from build123d import *

# Parameters (mm, degrees)
SKETCH1_W           = 109.86
SKETCH1_H           = 109.86
SKETCH1_R           = 4.25
BOSS_EXTRUDE1_DEPTH = 201
FILLET1_R           = 5
SKETCH2_R           = 27.6
BOSS_EXTRUDE2_DEPTH = 1.52
SKETCH3_R           = 9.5
BOSS_EXTRUDE3_DEPTH = 55.37
CUT_EXTRUDE1_START  = -12.5
CUT_EXTRUDE1_DEPTH  = 205.37
FILLET2_R           = 3


with BuildPart() as part:
    # Sketch1 → Boss-Extrude1 (new body)
    with BuildSketch(Plane(origin=(0, 0, 0), x_dir=(1, 0, 0), z_dir=(0, 1, 0))):
        Rectangle(SKETCH1_W, SKETCH1_H)
        with Locations(Location((-44.5, 44.5, 0), (0, 0, 270))):
            Circle(SKETCH1_R, mode=Mode.SUBTRACT)
        with Locations(Location((44.5, 44.5, 0), (0, 0, 270))):
            Circle(SKETCH1_R, mode=Mode.SUBTRACT)
        with Locations(Location((44.5, -44.5, 0), (0, 0, 270))):
            Circle(SKETCH1_R, mode=Mode.SUBTRACT)
        with Locations(Location((-44.5, -44.5, 0), (0, 0, 270))):
            Circle(SKETCH1_R, mode=Mode.SUBTRACT)
    extrude(amount=-BOSS_EXTRUDE1_DEPTH)

    # Fillet1
    fillet1_edges = [part.edges().sort_by_distance(p)[0] for p in [
        (54.93, -100.5, 54.93),
        (-54.93, -100.5, 54.93),
        (-54.93, -100.5, -54.93),
        (54.93, -100.5, -54.93),
    ]]
    fillet(fillet1_edges, radius=FILLET1_R)

    # Sketch2 → Boss-Extrude2 (add)
    with BuildSketch(Plane(origin=(0, 0, 0), x_dir=(1, 0, 0), z_dir=(0, 1, 0))):
        with Locations(Location((0, 0, 0), (0, 0, 90))):
            Circle(SKETCH2_R)
    extrude(amount=BOSS_EXTRUDE2_DEPTH)

    # Sketch3 → Boss-Extrude3 (add)
    with BuildSketch(Plane(origin=(0, 0, 0), x_dir=(1, 0, 0), z_dir=(0, 1, 0))):
        with Locations(Location((0, 0, 0), (0, 0, 270))):
            Circle(SKETCH3_R)
    extrude(amount=BOSS_EXTRUDE3_DEPTH)

    # Sketch5 → Cut-Extrude1 (cut)
    with BuildSketch(Plane(origin=(0, 0, 0), x_dir=(1, 0, 0), z_dir=(0, 1, 0)).offset(CUT_EXTRUDE1_START)):
        with BuildLine():
            Line((-44.5, 32.5), (-57.57926657, 32.5))
            Line((-57.57926657, 32.5), (-57.57926657, 62.356452686))
            Line((-57.57926657, 62.356452686), (-32.5, 61.861560204))
            Line((-32.5, 61.861560204), (-32.5, 44.5))
            ThreePointArc((-32.5, 44.5), (-36.014718626, 36.014718626), (-44.5, 32.5))
        make_face()
        with BuildLine():
            Line((62.356452686, 57.57926657), (61.861560204, 32.5))
            Line((61.861560204, 32.5), (44.5, 32.5))
            ThreePointArc((44.5, 32.5), (36.014718626, 36.014718626), (32.5, 44.5))
            Line((32.5, 44.5), (32.5, 57.57926657))
            Line((32.5, 57.57926657), (62.356452686, 57.57926657))
        make_face()
        with BuildLine():
            Line((57.57926657, -62.356452686), (32.5, -61.861560204))
            Line((32.5, -61.861560204), (32.5, -44.5))
            ThreePointArc((32.5, -44.5), (36.014718626, -36.014718626), (44.5, -32.5))
            Line((44.5, -32.5), (57.57926657, -32.5))
            Line((57.57926657, -32.5), (57.57926657, -62.356452686))
        make_face()
        with BuildLine():
            Line((-62.356452686, -57.57926657), (-61.861560204, -32.5))
            Line((-61.861560204, -32.5), (-44.5, -32.5))
            ThreePointArc((-44.5, -32.5), (-36.014718626, -36.014718626), (-32.5, -44.5))
            Line((-32.5, -44.5), (-32.5, -57.57926657))
            Line((-32.5, -57.57926657), (-62.356452686, -57.57926657))
        make_face()
    extrude(amount=-CUT_EXTRUDE1_DEPTH, mode=Mode.SUBTRACT)

    # Fillet2
    fillet2_edges = [part.edges().sort_by_distance(p)[0] for p in [
        (32.5, -106.75, 54.93),
        (32.5, -106.75, -54.93),
        (54.93, -106.75, -32.5),
        (-54.93, -106.75, -32.5),
        (-32.5, -106.75, -54.93),
        (-32.5, -106.75, 54.93),
        (-54.93, -106.75, 32.5),
        (54.93, -106.75, 32.5),
    ]]
    fillet(fillet2_edges, radius=FILLET2_R)


solid = part.part
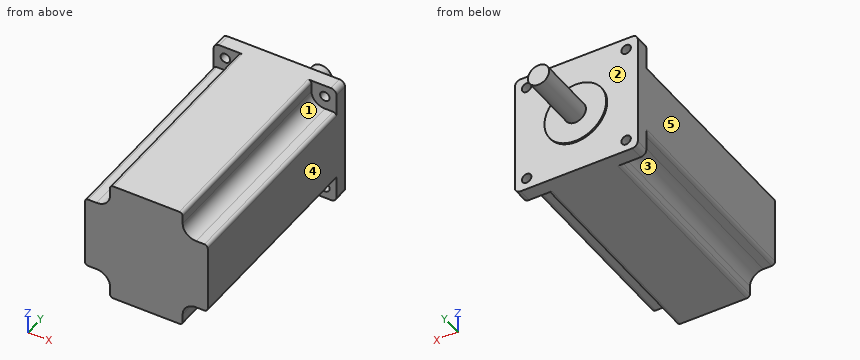
Geometry: final body of the model. Coordinates: model frame, mm. Face numbers are marked on the shaded views. A direction names the side the tool comes from. Coordinates: 2 decimals unless noted, no trailing zeros. Order: outer loops, then holes, each group sorted by start corner. A loop starts at its lowest first (then second) coordinate and runs counter-clockwise, first axis right, second up.
1) Section A-A (x = 0). Return loops of the section in (y, z).
Result sheet:
outline: (-201, -54.93) - (0, -54.93) - (0, -27.6) - (1.52, -27.6) - (1.52, -9.5) - (55.37, -9.5) - (55.37, 9.5) - (1.52, 9.5) - (1.52, 27.6) - (0, 27.6) - (0, 54.93) - (-201, 54.93) - close
2) Set-up query: the marked faces 1, 2, 3, 4 and 5. Return all of +Z, -Z, +X, -X, +Y, -Y with unobstructed straight access to the full face (end or side cutting, diameter ignored); none if empty.
Result sheet:
face 1: +Z, +X, -Y
face 2: +Y
face 3: -Z, -X, -Y
face 4: +Z, -Z, +X, +Y, -Y
face 5: +Z, -Z, -X, +Y, -Y
3) Section B-B (z = 0). Return loops of the section in (x, y).
Result sheet:
outline: (-54.93, -201) - (54.93, -201) - (54.93, 0) - (27.6, 0) - (27.6, 1.52) - (9.5, 1.52) - (9.5, 55.37) - (-9.5, 55.37) - (-9.5, 1.52) - (-27.6, 1.52) - (-27.6, 0) - (-54.93, 0) - close
4) Section D-D (z = 15). Return loops of the section in (x, y), then the cut area to 3 significant figures.
Result sheet:
outline: (-54.93, -201) - (54.93, -201) - (54.93, 0) - (23.17, 0) - (23.17, 1.52) - (-23.17, 1.52) - (-23.17, 0) - (-54.93, 0) - close
area: 22,200 mm2
5) Section C-C (y = -68.5). Return loops of the section in (x, z).
Result sheet:
outline: (-54.93, -29.5) arc R3 ccw to (-51.93, -32.5) - (-44.5, -32.5) arc R12 cw to (-32.5, -44.5) - (-32.5, -51.93) arc R3 ccw to (-29.5, -54.93) - (29.5, -54.93) arc R3 ccw to (32.5, -51.93) - (32.5, -44.5) arc R12 cw to (44.5, -32.5) - (51.93, -32.5) arc R3 ccw to (54.93, -29.5) - (54.93, 29.5) arc R3 ccw to (51.93, 32.5) - (44.5, 32.5) arc R12 cw to (32.5, 44.5) - (32.5, 51.93) arc R3 ccw to (29.5, 54.93) - (-29.5, 54.93) arc R3 ccw to (-32.5, 51.93) - (-32.5, 44.5) arc R12 cw to (-44.5, 32.5) - (-51.93, 32.5) arc R3 ccw to (-54.93, 29.5) - close
6) First-contact query: P1, Ø3.5, axis at y = -149, z = 49.5, coming from the +X side; P2, Ø12, axis at x = 3.5, z = 35.5, coming from the +Y side; P3, Ø8, axis at y = -149, z = -47, coming from the -X side. Flat tips, straight axial feed; report the tip coordinate or a pass-through.
Result sheet:
P1: stops at x = 32.5
P2: stops at y = 0
P3: stops at x = -32.59
7) Ray query, probe 1 along X at (y, z) = (-7.25, -44.5); probe 2 along Z at (x, y) = (44, -8); probe 3 along Y at (x, z) = (40, -23.5). Return the intervals inside material, ascending.
Result sheet:
probe 1: x = -54.93 to -48.75, -40.25 to 40.25, 48.75 to 54.93
probe 2: z = -54.93 to -48.72, -40.28 to 40.28, 48.72 to 54.93
probe 3: y = -201 to 0
